Study the drawing (mm; zero at the part's minimum x, y, z) and answer. A direction names the side the tool comes from. Coordinates: 2 decimals unless noted, no trailing zeros. Loops run counter-clockwise (first coordinate to the right, second up) from the corner with the lowest first, then second, coordinate; pieces in that order, holes last. Notation, with made-up numbers: M 55,11.25 L 87,11.25 A20 cw 87,37.25 Z; hole C -22,35.5 d1. An arc over 180 degrees is marked long. Use one line per item in the form item = value. Start each with the question number.
1. Flat-ended cylindrical pins translate along their axes: pin 1 (3 mm diameter, centred on x = 30, y = 7.5, fed in from -Z); pin 2 (3.5 mm diameter, centred on y = 3, z = 25.5, fed in from +X); pin 3 (5.5 mm diameter, centred on x = 39, y = 2, fed in from +Z). Find the tip coordinate at first contact, or state that the pin passes through.
2. The part is cut by section A-A (y = 1). Give the vertices of the cut face in (x, z).
3. The part is cut by section B-B (z = 11.25). Give the vertices of the cut face in (x, y), plus the area to 3 significant figures.
4. A tool of negligible diameter and unlimited length cuts with its end or side. For the marked faces 5, 6 and 7, from which of +Z, -Z, +X, -X, +Y, -Y can it reach the whole face along a straight path? Write none if from no direction.
5. For a pull along X with two mould halves and no side action, classify the marked faces 1, 2, 3 and 4 as released by +X, released by -X, zero draft, split by the parting line, or undercut.
6. Find the intervals of material crossed by probe 1 along Z at (x, y) = (19, 2.5); probe 2 along Z at (x, y) = (33, 1); probe 3 along Z at (x, y) = (52.5, 7.5), in increasing order. Write a range as [from, to].
7. The part is cut by section D-D (y = 5.75). Give the vertices of the cut face in (x, z).
8. The part is cut by section C-C (x = 28). Give the vertices of the cut face in (y, z).
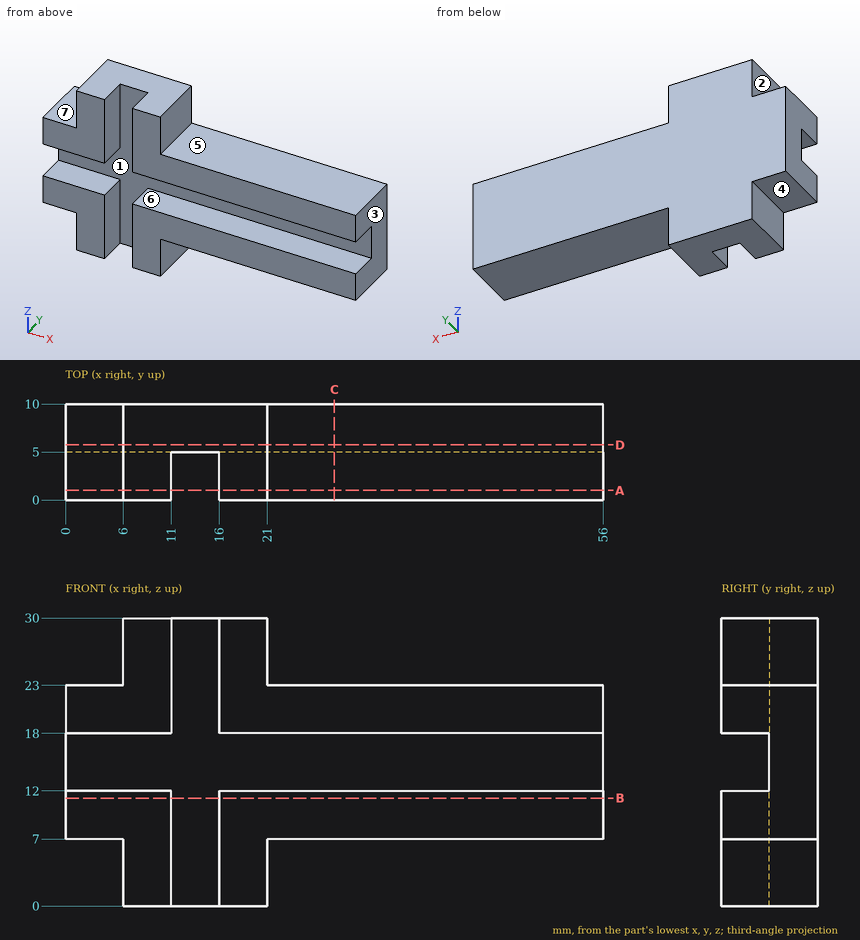
Computed values:
q1.pin_1 = 7
q1.pin_2 = 21
q1.pin_3 = 23
q2.outline = M 0,7 L 6,7 L 6,0 L 11,0 L 11,12 L 0,12 Z; M 0,18 L 11,18 L 11,30 L 6,30 L 6,23 L 0,23 Z; M 16,0 L 21,0 L 21,7 L 56,7 L 56,12 L 16,12 Z; M 16,18 L 56,18 L 56,23 L 21,23 L 21,30 L 16,30 Z
q3.outline = M 0,0 L 11,0 L 11,5 L 16,5 L 16,0 L 56,0 L 56,10 L 0,10 Z
q3.area = 535 mm²
q4.face_5 = +Z, +X, +Y, -Y
q4.face_6 = +X, -X, -Y
q4.face_7 = +Z, -X, +Y, -Y
q5.face_1 = undercut
q5.face_2 = released by -X
q5.face_3 = released by +X
q5.face_4 = zero draft
q6.probe_1 = [0, 12], [18, 30]
q6.probe_2 = [7, 12], [18, 23]
q6.probe_3 = [7, 23]
q7.outline = M 0,7 L 6,7 L 6,0 L 21,0 L 21,7 L 56,7 L 56,23 L 21,23 L 21,30 L 6,30 L 6,23 L 0,23 Z
q8.outline = M 0,7 L 10,7 L 10,23 L 0,23 L 0,18 L 5,18 L 5,12 L 0,12 Z
